from build123d import *

# Parameters (mm, degrees)
SKETCH1_W                  = 241.3
SKETCH1_H                  = 38.1
BOSS_EXTRUDE1_DEPTH        = 2.54
SKETCH2_R                  = 2.54
CUT_EXTRUDE1_DEPTH         = 2.54
LPATTERN1_COUNT            = 19
LPATTERN1_PITCH            = 12.7
SKETCHED_START             = -120.65
SKETCHED_BEND2_OUTLINE_W   = 2.54
SKETCHED_BEND2_OUTLINE_H   = 38.1
SKETCHED_BEND2_DEPTH       = 23.699379955
SKETCHED_START_2           = -96.631937929
SKETCHED_BEND2_2_OUTLINE_W = 24.560620045
SKETCHED_BEND2_2_OUTLINE_H = 38.1
SKETCHED_BEND2_2_OUTLINE_R = 2.54
SKETCHED_BEND2_2_DEPTH     = 2.221317884
SKETCHED_START_3           = -96.950620045
SKETCHED_BEND2_3_OUTLINE_W = 24.560620045
SKETCHED_BEND2_3_OUTLINE_H = 38.1
SKETCHED_BEND2_3_OUTLINE_R = 2.54
SKETCHED_BEND2_3_DEPTH     = 3.2766
SKETCHED_START_4           = -20
SKETCHED_BEND2_4_DEPTH     = 40
SKETCHED_START_5           = 96.950620045
SKETCHED_BEND3_OUTLINE_W   = 2.54
SKETCHED_BEND3_OUTLINE_H   = 38.1
SKETCHED_BEND3_DEPTH       = 23.699379955
SKETCHED_START_6           = 94.410620045
SKETCHED_BEND3_2_OUTLINE_W = 24.560620045
SKETCHED_BEND3_2_OUTLINE_H = 38.1
SKETCHED_BEND3_2_OUTLINE_R = 2.54
SKETCHED_BEND3_2_DEPTH     = 2.221317884
SKETCHED_START_7           = 93.674020045
SKETCHED_BEND3_3_OUTLINE_W = 24.560620045
SKETCHED_BEND3_3_OUTLINE_H = 38.1
SKETCHED_BEND3_3_OUTLINE_R = 2.54
SKETCHED_BEND3_3_DEPTH     = 3.2766
SKETCHED_BEND3_4_DEPTH     = 40


with BuildPart() as part:
    # Sketch1 → Boss-Extrude1 (new body)
    with BuildSketch(Plane(origin=(0, 0, 0), x_dir=(1, 0, 0), z_dir=(0, 1, 0))):
        Rectangle(SKETCH1_W, SKETCH1_H)
    extrude(amount=BOSS_EXTRUDE1_DEPTH)

    # Sketch2 → Cut-Extrude1 (cut)
    with BuildSketch(Plane(origin=(0, 2.54, 0), x_dir=(1, 0, 0), z_dir=(0, 1, 0))):
        with Locations(Location((-114.3, 0, 0), (0, 0, 270))):
            Circle(SKETCH2_R)
    cut_extrude1 = extrude(amount=-CUT_EXTRUDE1_DEPTH, mode=Mode.SUBTRACT)

    # LPattern1: Cut-Extrude1 ×19
    with Locations(*[(i * LPATTERN1_PITCH, 0, 0) for i in range(1, LPATTERN1_COUNT)]):
        add(cut_extrude1, mode=Mode.SUBTRACT)

    # Sketched Bend2: read off the stored shape, not the designer's step
    # Sketched Bend2 outline → Sketched Bend2 (cut)
    with BuildSketch(Plane.YZ.offset(SKETCHED_START)):
        with Locations((1.27, 0)):
            Rectangle(SKETCHED_BEND2_OUTLINE_W, SKETCHED_BEND2_OUTLINE_H)
    extrude(amount=SKETCHED_BEND2_DEPTH, mode=Mode.SUBTRACT)

    # Sketched Bend2 2 outline → Sketched Bend2 2 (add)
    with BuildSketch(Plane.YZ.offset(SKETCHED_START_2)):
        with Locations((14.820310023, 0)):
            Rectangle(SKETCHED_BEND2_2_OUTLINE_W, SKETCHED_BEND2_2_OUTLINE_H)
        with Locations((8.050620045, 0)):
            Circle(SKETCHED_BEND2_2_OUTLINE_R, mode=Mode.SUBTRACT)
        with Locations((20.750620045, 0)):
            Circle(SKETCHED_BEND2_2_OUTLINE_R, mode=Mode.SUBTRACT)
    extrude(amount=SKETCHED_BEND2_2_DEPTH)

    # Sketched Bend2 3 outline → Sketched Bend2 3 (add)
    with BuildSketch(Plane.YZ.offset(SKETCHED_START_3)):
        with Locations((14.820310023, 0)):
            Rectangle(SKETCHED_BEND2_3_OUTLINE_W, SKETCHED_BEND2_3_OUTLINE_H)
        with Locations((8.050620045, 0)):
            Circle(SKETCHED_BEND2_3_OUTLINE_R, mode=Mode.SUBTRACT)
        with Locations((20.750620045, 0)):
            Circle(SKETCHED_BEND2_3_OUTLINE_R, mode=Mode.SUBTRACT)
    extrude(amount=SKETCHED_BEND2_3_DEPTH)

    # Sketched Bend2 4 outline → Sketched Bend2 4 (cut)
    with BuildSketch(Plane.XY.offset(SKETCHED_START_4)):
        with BuildLine():
            Line((-93.674020045, 27.100620045), (-94.410620045, 27.100620045))
            Line((-94.410620045, 27.100620045), (-94.410620045, 3.2766))
            ThreePointArc((-94.410620045, 3.2766), (-94.1948749, 2.755745145), (-93.674020045, 2.54))
            Line((-93.674020045, 2.54), (-93.674020045, 27.100620045))
        make_face()
        with BuildLine():
            ThreePointArc((-93.674020045, 0), (-95.990926125, 0.95969392), (-96.950620045, 3.2766))
            Line((-96.950620045, 3.2766), (-96.950620045, 0))
            Line((-96.950620045, 0), (-93.674020045, 0))
        make_face()
    extrude(amount=SKETCHED_BEND2_4_DEPTH, mode=Mode.SUBTRACT)

    # Sketched Bend3: read off the stored shape, not the designer's step
    # Sketched Bend3 outline → Sketched Bend3 (cut)
    with BuildSketch(Plane.YZ.offset(SKETCHED_START_5)):
        with Locations((1.27, 0)):
            Rectangle(SKETCHED_BEND3_OUTLINE_W, SKETCHED_BEND3_OUTLINE_H)
    extrude(amount=SKETCHED_BEND3_DEPTH, mode=Mode.SUBTRACT)

    # Sketched Bend3 2 outline → Sketched Bend3 2 (add)
    with BuildSketch(Plane.YZ.offset(SKETCHED_START_6)):
        with Locations((14.820310023, 0)):
            Rectangle(SKETCHED_BEND3_2_OUTLINE_W, SKETCHED_BEND3_2_OUTLINE_H)
        with Locations((8.050620045, 0)):
            Circle(SKETCHED_BEND3_2_OUTLINE_R, mode=Mode.SUBTRACT)
        with Locations((20.750620045, 0)):
            Circle(SKETCHED_BEND3_2_OUTLINE_R, mode=Mode.SUBTRACT)
    extrude(amount=SKETCHED_BEND3_2_DEPTH)

    # Sketched Bend3 3 outline → Sketched Bend3 3 (add)
    with BuildSketch(Plane.YZ.offset(SKETCHED_START_7)):
        with Locations((14.820310023, 0)):
            Rectangle(SKETCHED_BEND3_3_OUTLINE_W, SKETCHED_BEND3_3_OUTLINE_H)
        with Locations((8.050620045, 0)):
            Circle(SKETCHED_BEND3_3_OUTLINE_R, mode=Mode.SUBTRACT)
        with Locations((20.750620045, 0)):
            Circle(SKETCHED_BEND3_3_OUTLINE_R, mode=Mode.SUBTRACT)
    extrude(amount=SKETCHED_BEND3_3_DEPTH)

    # Sketched Bend3 4 outline → Sketched Bend3 4 (cut)
    with BuildSketch(Plane.XY.offset(SKETCHED_START_4)):
        with BuildLine():
            Line((96.950620045, 0), (96.950620045, 3.2766))
            ThreePointArc((96.950620045, 3.2766), (95.990926125, 0.95969392), (93.674020045, 0))
            Line((93.674020045, 0), (96.950620045, 0))
        make_face()
        with BuildLine():
            ThreePointArc((93.674020045, 2.54), (94.1948749, 2.755745145), (94.410620045, 3.2766))
            Line((94.410620045, 3.2766), (94.410620045, 27.100620045))
            Line((94.410620045, 27.100620045), (93.674020045, 27.100620045))
            Line((93.674020045, 27.100620045), (93.674020045, 2.54))
        make_face()
    extrude(amount=SKETCHED_BEND3_4_DEPTH, mode=Mode.SUBTRACT)


solid = part.part
Verification items for the finished model (mm, model axes). A direction names the side the tool comes from. Coordinates: 2 decimals unless noted, no trailing zeros. Order: outer loops, then holes, each group sorted by start corner. A loop starts at its lowest first (then second) coordinate and runs counter-clockwise, first axis right, second up. Notation, with made-up numbers: (78.25, -37) -> (87.25, -37) arc R21 cw to (87.25, -14) -> close; hole circle Ø1 at (24.25, 71.5). An arc over 180 degrees is marked (long way). Use CSV: the item, a comma, the result in double quotes. Start each with the question number.
Q1. Thickness scan on line 1 along X through (y, z) = (24, -17); line 2 along Z through (x, y) = (63.5, 1.3); line 3 along Y through (x, z) = (-17, 0). Record the ranges inside material, lowest first.
Q2. Depth check by flat-ended pin: P1, Ø6.5, axis at x = 25.4, z = 0, coming from the +Y side; P2, Ø4.5, axis at x = 88.9, z = 0, coming from the -Y side. Enter the tip coordinate at first touch or a pass-through.
Q3. Section check B-B, the plane y = 16.5. Record the cut outline in (x, z), and give its area (3 significant figures).
Q4. Section check A-A, the plane x = -88.9. Record the cut outline in (y, z).
Q5. Tool access check on faces 1 (the flat face through (-1, 2.54, -5)), 2 (the cylindrical face through (-27.88, 1.29, -0.55)). Record the directions out of +Z, -Z, +X, -X, +Y, -Y that give a thin tool (end or side, any length) a straight path to the whole face; none if there is none.
Q6. Section check D-D, the plane x = -31.5. Record the cut outline in (y, z).
Q7. Draft check along X on faces 3 (the cylindrical face through (73.72, 1.29, -0.55)), 4 (the cylindrical face through (-48.28, 1.29, -0.33)), 5 (the cylindrical face through (96.02, 0.99, -0.27)), 6 (the flat face through (0, 1, -19.05)). Enter one of: +X half, -X half, draft (parallel to the pull), parting line (faces both ways), or undercut.
Q8. Section check C-C, the plane z = 7. Record the cut outline in (x, y), and give its area (3 significant figures).
Returned:
1,line 1,"x = -96.95 to -94.41, 94.41 to 96.95"
1,line 2,"z = -19.05 to -2.54, 2.54 to 19.05"
1,line 3,"y = 0 to 2.54"
2,P1,"stops at y = 2.54"
2,P2,"passes through"
3,outline,"(-96.95, -19.05) -> (-94.41, -19.05) -> (-94.41, 19.05) -> (-96.95, 19.05) -> close; (94.41, -19.05) -> (96.95, -19.05) -> (96.95, 19.05) -> (94.41, 19.05) -> close"
3,area,"194 mm^2"
4,outline,"(0, -19.05) -> (2.54, -19.05) -> (2.54, -2.54) -> (0, -2.54) -> close; (0, 2.54) -> (2.54, 2.54) -> (2.54, 19.05) -> (0, 19.05) -> close"
5,face 1,"+Z, -Z, +Y"
5,face 2,"+Y, -Y"
6,outline,"(0, -19.05) -> (2.54, -19.05) -> (2.54, 19.05) -> (0, 19.05) -> close"
7,face 3,"undercut"
7,face 4,"undercut"
7,face 5,"+X half"
7,face 6,"draft"
8,outline,"(-96.95, 3.28) arc R3.28 ccw to (-93.67, 0) -> (93.67, 0) arc R3.28 ccw to (96.95, 3.28) -> (96.95, 27.1) -> (94.41, 27.1) -> (94.41, 3.28) arc R0.74 cw to (93.67, 2.54) -> (-93.67, 2.54) arc R0.74 cw to (-94.41, 3.28) -> (-94.41, 27.1) -> (-96.95, 27.1) -> close"
8,area,"613 mm^2"
